Autodesk Inventor part; units mm, degrees
ref_plane "YZ Plane" through (0, 0, 0) normal (1, 0, 0) x (0, 1, 0)
ref_plane "XZ Plane" through (0, 0, 0) normal (0, 1, 0) x (-1, 0, 0)
ref_plane "XY Plane" through (0, 0, 0) normal (0, 0, 1) x (1, 0, 0)
sketch "Sketch1" plane through (0, 0, 0) normal (0, 0, 1) x (1, 0, 0)
  line L0 (5.375, 4) -> (5.375, 1.25)
  line L1 (5.375, 1.25) -> (-0.125, 1.25)
  line L2 (-0.125, 1.25) -> (-0.125, -1.25)
  line L3 (-0.125, -1.25) -> (5.375, -1.25)
  line L4 (5.375, -1.25) -> (5.375, -4)
  line L5 (5.375, -4) -> (-5.375, -4)
  line L6 (-5.375, -4) -> (-5.375, 4)
  line L7 (-5.375, 4) -> (5.375, 4)
  line L8 (-12.6672, 0) -> (12.6672, 0) construction
  line L9 (0, 8.1446) -> (0, -8.1446) construction
  point P0 (0, 0)
  point P1 (0, 0)
  dimension "d1" = 8
  dimension "d2" = 10.75
  dimension "d4" = 2.5
  dimension "d7" = 0.125
extrude "Extrusion1" add sketch "Sketch1" along normal mid plane 2.5
properties part number "pitahaya5"
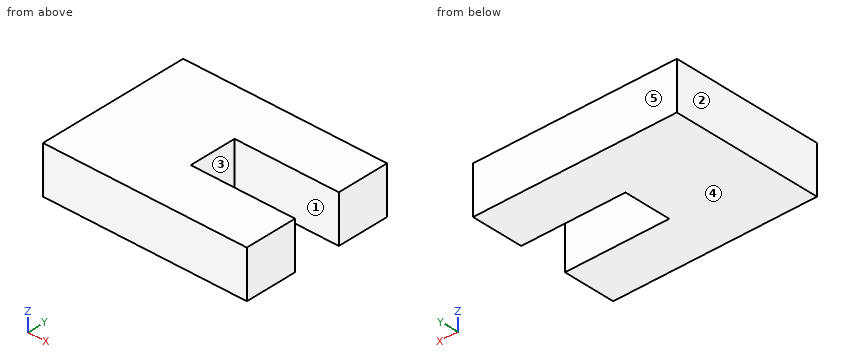
Read the model definition and answer for the solid it produces. Units are mm, in the model's axes. Face numbers are marked on the shaded views. A direction names the side the tool comes from. Give positions to 0.01 mm unless a question says otherwise; leave off trailing zeros. Loops run counter-clockwise (first coordinate to the right, second up) from the corner with the lowest first, then second, coordinate; pieces in that order, holes last. Notation, with made-up numbers: (15.5, -24.75) -> (73.5, -24.75) arc R6 cw to (73.5, -19.75) -> close; hole circle Ø10 at (51, -10.75). An arc over 180 degrees is marked (long way). Use a Markdown table: item, result.
Q1. Section B-B, the plane z = -0.65 is taken. Determine the outline of the cut face in (x, y) (3 decimals).
Solved:
| item | result |
|---|---|
| outline | (-5.375, -4) -> (5.375, -4) -> (5.375, -1.25) -> (-0.125, -1.25) -> (-0.125, 1.25) -> (5.375, 1.25) -> (5.375, 4) -> (-5.375, 4) -> close |
Q2. Determine the mould class of the marked faces 3, 4 and 5 for opening direction Y: pulls with the +Y half, pulls with the -Y half, needs draft (parallel to the pull), parting line crosses it, or undercut.
Solved:
| item | result |
|---|---|
| face 3 | undercut |
| face 4 | needs draft |
| face 5 | pulls with the +Y half |
Q3. Section A-A, the plane x = 4.5 is taken. Determine the outline of the cut face in (y, z), then the cut area to 4 significant figures.
Solved:
| item | result |
|---|---|
| outline | (-4, -1.25) -> (-1.25, -1.25) -> (-1.25, 1.25) -> (-4, 1.25) -> close; (1.25, -1.25) -> (4, -1.25) -> (4, 1.25) -> (1.25, 1.25) -> close |
| area | 13.75 mm^2 |
Q4. A tool of negligible diameter and unlimited length cuts with its end or side. For the marked faces 1 and 2, from which of +Z, -Z, +X, -X, +Y, -Y can it reach the whole face along a straight path? Write none if from no direction.
Solved:
| item | result |
|---|---|
| face 1 | +Z, -Z, +X |
| face 2 | +Z, -Z, -X, +Y, -Y |
Q5. Find the intervals of material crossed by line 1 along Y through (x, z) = (0, -0.15); line 2 along X through (y, z) = (0.75, 0.45) (3 decimals), in increasing order.
Solved:
| item | result |
|---|---|
| line 1 | y = -4 to -1.25, 1.25 to 4 |
| line 2 | x = -5.375 to -0.125 |
Q6. This flat-tipped pin is pushed along its axis until it touches: pin 1 (0.8 mm diameter, centred on y = 0, z = 0, fed in from +X) (3 decimals). Where does it stop, or does it pass through?
Solved:
| item | result |
|---|---|
| pin 1 | stops at x = -0.125 |
